Build history of the part. All positions in model axes, mm. Face numbers are marked on the shaded views. A direction names the side the tool comes from. Coordinates: 2 decimals unless noted, no trailing zeros. Loops run counter-clockwise (first coordinate to the right, second up) from the corner with the lowest first, then second, coordinate; pieces in that order, holes last.
Item 1: Cut at C-C (x = -17). List the corners of the cut face in (y, z), and give its area (3 significant figures).
Item 2: Flat gauge pins, fed straight in: pin 1 (8.5 mm diameter, centred on y = 40.5, z = 7.5, fed in from +X); pin 2 (3 mm diameter, centred on x = 0.01, z = 7.6, fed in from +Y); pin 3 (12 mm diameter, centred on x = 5.5, y = 35, fed in from +Z); pin 4 (0.9 mm diameter, centred on y = -38.5, z = 14, fed in from +X). Where does each tip first touch, or does it go through?
Item 3: Cut at D-D (x = 1). List the corners of the cut face in (y, z).
Item 4: Cut at B-B (z = 13.25). List the corners of the cut face in (x, y).
Item 5: Drill centre lines: line 1 along Y through (x, z) = (16, 8); line 2 along Y through (x, z) = (-20.5, 11.5); line 3 along X through (y, z) = (-13, 15.25). Where is each one in solid material? Low to high.
Item 6: 3-axis set-ups, long thin cutter, end or side, ignore diameter. For the marked faces 1, 2 and 3: which of +Z, -Z, +X, -X, +Y, -Y reach the whole face in a straight line?
Item 7: Cut at A-A (y = 0). List the corners of the cut face in (x, z), and give its area (3 significant figures).
Item 8: Mould opens along Y. For the marked faces 4, 5 and 6 say: released by +Y, released by -Y, zero draft, split by the parting line, or undercut.
Autodesk Fusion 360 part; units mm, degrees
sketch "Skizze1" plane through (0, 0, 0) normal (0, 0, 1) x (1, 0, 0)
  circle A0 centre (0, 0) radius 35
  circle A1 centre (0, 0) radius 40
  line L0 (10, 30) -> (-10, 30)
  line L1 (-10, 30) -> (-10, 45)
  line L2 (-10, 45) -> (10, 45)
  line L3 (10, 45) -> (10, 30)
  line L4 (15, 35) -> (10, 35)
  line L5 (10, 35) -> (10, 45)
  line L6 (10, 45) -> (15, 45)
  line L7 (15, 45) -> (15, 35)
  line L8 (-10, 35) -> (-15, 35)
  line L9 (-15, 35) -> (-15, 45)
  line L10 (-15, 45) -> (-10, 45)
  line L11 (-10, 45) -> (-10, 35)
  line L12 (-15, -35) -> (15, -35)
  line L13 (15, -35) -> (15, -40)
  line L14 (15, -40) -> (-15, -40)
  line L15 (-15, -40) -> (-15, -35)
  dimension "d1" = 70
  dimension "d2" = 80
extrude "Extrusion1" add sketch "Skizze1" along normal blind 25 contours A0 A1 L3 L4 L7 L12 L13 | A0 A1 L1 L8 L9 L12 L15 | A1 L12 L13 L15 | A1 L3 L4 L5 L7 | A1 L1 L8 L9 L11 | A1 L3 L5 L6 L7 | A1 L14 L15 | A1 L13 L14 | A1 L1 L9 L10 L11
hole "Bohrung1" at (-0.0001, -40, 17.6541) direction (0, 1, 0) diameter 5 depth 15 tip angle 118
hole "Bohrung2" at (0.0132, -40, 7.6012) direction (0, 1, 0) diameter 5 depth 15 tip angle 118
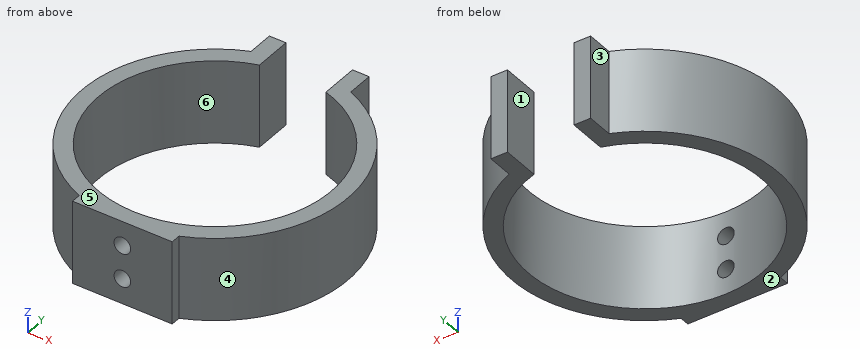
Filled sheet:
1. outline: (-36.21, 0) - (-30.59, 0) - (-30.59, 25) - (-36.21, 25) - close; (30.59, 0) - (36.21, 0) - (36.21, 25) - (30.59, 25) - close
1. area: 281 mm2
2. pin 1: stops at x = 16.91
2. pin 2: passes through
2. pin 3: stops at z = 25
2. pin 4: stops at x = 15
3. outline: (-40, 0) - (-34.99, 0) - (-34.99, 5.3) - (-40, 5.3) - close; (-40, 9.9) - (-34.99, 9.9) - (-34.99, 15.36) - (-40, 15.36) - close; (-40, 19.95) - (-34.99, 19.95) - (-34.99, 25) - (-40, 25) - close
4. outline: (-15, -40) - (15, -40) - (15, -37.08) arc R40 ccw to (15, 37.08) - (15, 45) - (10, 45) - (10, 33.54) arc R35 cw (long way) to (-10, 33.54) - (-10, 45) - (-15, 45) - (-15, 37.08) arc R40 ccw to (-15, -37.08) - close
5. line 1: y = -36.66 to -31.13, 31.13 to 36.66
5. line 2: y = -34.35 to -28.37, 28.37 to 34.35
5. line 3: x = -37.83 to -32.5, 32.5 to 37.83
6. face 1: +Z, -Z, +Y
6. face 2: -Z, +X, -X, +Y, -Y
6. face 3: +Z, -Z, -X, +Y
7. outline: (-40, 0) - (-35, 0) - (-35, 25) - (-40, 25) - close; (35, 0) - (40, 0) - (40, 25) - (35, 25) - close
7. area: 250 mm2
8. face 4: split by the parting line
8. face 5: zero draft
8. face 6: undercut
